```python
from build123d import *

# Parameters (mm, degrees)
BOSS_EXTRUDE1_DEPTH = 50
SKETCH2_W           = 55.7
SKETCH2_H           = 36
SKETCH2_R           = 2.55
BOSS_EXTRUDE2_DEPTH = 2


with BuildPart() as part:
    # Sketch1 → Boss-Extrude1 (new body)
    with BuildSketch(Plane(origin=(0, 0, 0), x_dir=(0, 0, -1), z_dir=(1, 0, 0))):
        Polygon((0, 10), (0, 0), (6, 0), (6, 4.0875), (4, 4.0875), (4, 2.5), (2, 2.5), (2, 7.5), (4, 7.5), (4, 5.9125), (6, 5.9125), (6, 10), align=None)
    extrude(amount=BOSS_EXTRUDE1_DEPTH)

    # Sketch2 → Boss-Extrude2 (add)
    with BuildSketch(Plane(origin=(0, 10, 0), x_dir=(1, 0, 0), z_dir=(0, 1, 0))):
        with Locations((25, 3)):
            Rectangle(SKETCH2_W, SKETCH2_H)
        with Locations(Location((5.15, 13, 0), (0, 0, 270))):
            Circle(SKETCH2_R, mode=Mode.SUBTRACT)
        with Locations(Location((44.85, 13, 0), (0, 0, 270))):
            Circle(SKETCH2_R, mode=Mode.SUBTRACT)
        with Locations(Location((44.85, -7, 0), (0, 0, 270))):
            Circle(SKETCH2_R, mode=Mode.SUBTRACT)
        with Locations(Location((5.15, -7, 0), (0, 0, 270))):
            Circle(SKETCH2_R, mode=Mode.SUBTRACT)
    extrude(amount=BOSS_EXTRUDE2_DEPTH)


solid = part.part
```
For this review, take the finished solid that the model builds, in its own axes (mm). A direction names the side the tool comes from. Coordinates: 2 decimals unless noted, no trailing zeros. Write each loop counter-clockwise with the first axis right and the second up, starting at its lowest first coordinate (ties: lowest second). Pieces come first, ordered by that corner, then holes.
(1) Add section D-D on z = -1. Give the boundary of the cut face in (x, y), then the cut area to 3 significant figures.
(2) Add section B-B on z = 7. Give the boundary of the cut face in (x, y), then the cut area to 3 significant figures.
(3) The part is to be moulded in two halves that separate along Y. For faces 4 (the face through (25, 4.088, -5)), 5 (the face through (-2.85, 11, -3)), 6 (the face through (25, 0, -3)), say which applies: +Y half, -Y half, draft (parallel to the pull), parting line (faces both ways), or undercut.
(4) For pin 1 Ø5.5 at (x, y) = (15, 6) entering from -Z; pin 2 Ø8 at (x, z) = (44.85, 7) entering from -Y; pin 3 Ø0.8 at (x, y) = (22, 6.5) entering from +Z, all flat-tipped, find the tip position at first contact; note any pin that passes through.
(5) Add section C-C on x = 33. Give the boundary of the cut face in (y, z).
(6) Tool access review of faces 1 (the face through (25, 5.912, -5)), 2 (the face through (25, 7, -4)), 3 (the face through (25, 8, -6)): name each direction out of +Z, -Z, +X, -X, +Y, -Y from which nothing blocks a thin tool from reaching the whole face with its end or side.
(7) Add section A-A on x = 5.15. Give the boundary of the cut face in (y, z), then the cut area to 4 significant figures.
(8) Wall thickness on probe 1 along X at (y, z) = (10.75, -13); probe 2 along Z at (x, y) = (18, 7); probe 3 along Z at (x, y) = (48.5, 5.75): over which ranges is each line inside the solid? List them lowest first.
Answer sheet:
1. outline: (-2.85, 10) - (0, 10) - (0, 0) - (50, 0) - (50, 10) - (52.85, 10) - (52.85, 12) - (-2.85, 12) - close
1. area: 611 mm2
2. outline: (-2.85, 10) - (2.6, 10) - (2.6, 12) - (-2.85, 12) - close; (7.7, 10) - (42.3, 10) - (42.3, 12) - (7.7, 12) - close; (47.4, 10) - (52.85, 10) - (52.85, 12) - (47.4, 12) - close
2. area: 91.0 mm2
3. face 4: undercut
3. face 5: draft
3. face 6: -Y half
4. pin 1: stops at z = -6
4. pin 2: stops at y = 10
4. pin 3: stops at z = 0
5. outline: (0, -6) - (4.09, -6) - (4.09, -4) - (2.5, -4) - (2.5, -2) - (7.5, -2) - (7.5, -4) - (5.91, -4) - (5.91, -6) - (10, -6) - (10, -21) - (12, -21) - (12, 15) - (10, 15) - (10, 0) - (0, 0) - close
6. face 1: -Z, +X, -X
6. face 2: +X, -X
6. face 3: -Z, +X, -X, -Y
7. outline: (0, -6) - (4.09, -6) - (4.09, -4) - (2.5, -4) - (2.5, -2) - (7.5, -2) - (7.5, -4) - (5.91, -4) - (5.91, -6) - (10, -6) - (10, -10.45) - (12, -10.45) - (12, 4.45) - (10, 4.45) - (10, 0) - (0, 0) - close; (10, -21) - (12, -21) - (12, -15.55) - (10, -15.55) - close; (10, 9.55) - (12, 9.55) - (12, 15) - (10, 15) - close
7. area: 97.95 mm2
8. probe 1: x = -2.85 to 2.6, 7.7 to 42.3, 47.4 to 52.85
8. probe 2: z = -6 to -4, -2 to 0
8. probe 3: z = -2 to 0
